Source: three-view drawing plus pictorial views. Frame: mm from the lowest corner of the part. A direction names the side the tool comes from. Round coordinates to 2 decimals unless told otherwise and drop trailing zeros. Loops run counter-clockwise (first coordinate to the right, second up) from the corner with the lowest first, then second, coordinate; pieces in that order, holes last. Notation, with made-up numbers: (58, 12.5) -> (112, 12.5) arc R22 ccw to (112, 48.5) -> close; hole circle Ø5 at (88.5, 9.5). An arc over 180 degrees is marked (long way). Answer in a Markdown table with one row per item. Add a question column.
Q1. Pin query (flat end, axial travel): pin 1 (4 mm diameter, centred on x = 53, z = 24, fed in from -Y); pin 2 (9 mm diameter, centred on x = 35, z = 41, fed in from +Y). Return the tip coordinate at first contact, or that it passes through.
Q2. Ray query, L1, parallel to X at y = 5, z = 48; L2, parallel to Z at x = 26.5, y = 17.25; L3, parallel to Y at x = 65, z = 3. Return the intervals inside material, ascending. Write a range as from..to.
Q3. Mould query, pull axis Z, two halves, no side actions, for the marked faces 3, 4 and 5. Classes: pulls with the +Z half, pulls with the -Z half, needs draft (parallel to the pull), parting line crosses it, or undercut.
Q4. Section D-D, the plane y = 20. Output: boundary loops of the cut face in (x, z), and give its area (3 significant figures).
Q5. Section B-B, the plane z = 11. Output: boundary loops of the cut face in (x, y), and give its area (3 significant figures).
Q6. Section C-C, the plane x = 23. Output: boundary loops of the cut face in (y, z).
Q7. Reachability of the marked faces 1 and 2 from +Z, -Z, +X, -X, +Y, -Y: full face, straight path, thin tool, end or side. Return the list, or none.
Q8. Section A-A, the plane y = 15.25. Output: boundary loops of the cut face in (x, z).
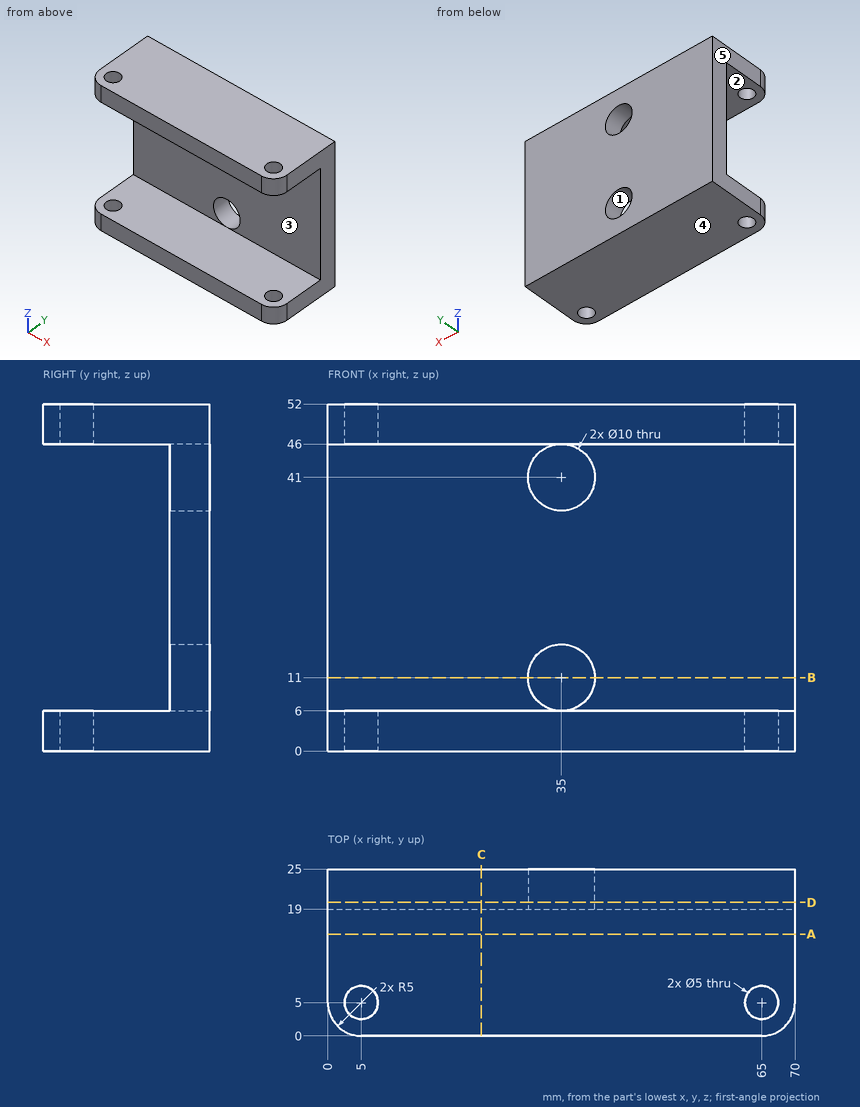
Answer block:
| question | item | result |
|---|---|---|
| 1 | pin 1 | y = 19 |
| 1 | pin 2 | through |
| 2 | L1 | 0..2.5, 7.5..62.5, 67.5..70 |
| 2 | L2 | 0..6, 46..52 |
| 2 | L3 | 0..2.5, 7.5..25 |
| 3 | face 3 | undercut |
| 3 | face 4 | pulls with the -Z half |
| 3 | face 5 | needs draft |
| 4 | outline | (0, 0) -> (70, 0) -> (70, 52) -> (0, 52) -> close; hole circle Ø10 at (35, 11); hole circle Ø10 at (35, 41) |
| 4 | area | 3,480 mm^2 |
| 5 | outline | (0, 19) -> (30, 19) -> (30, 25) -> (0, 25) -> close; (40, 19) -> (70, 19) -> (70, 25) -> (40, 25) -> close |
| 5 | area | 360 mm^2 |
| 6 | outline | (0, 0) -> (25, 0) -> (25, 52) -> (0, 52) -> (0, 46) -> (19, 46) -> (19, 6) -> (0, 6) -> close |
| 7 | face 1 | +Y, -Y |
| 7 | face 2 | +X, -X, -Y |
| 8 | outline | (0, 0) -> (70, 0) -> (70, 6) -> (0, 6) -> close; (0, 46) -> (70, 46) -> (70, 52) -> (0, 52) -> close |
